```python
from build123d import *

# Parameters (mm, degrees)
SKETCH2_R          = 2
CUT_EXTRUDE1_DEPTH = 41.551456831


with BuildPart() as part:
    # Sketch1 → Revolve1 (revolve)
    with BuildSketch(Plane.XY, mode=Mode.PRIVATE) as revolve1_sk:
        with BuildLine():
            ThreePointArc((5, -39.32455532), (3.535533906, -35.789021414), (0, -34.32455532))
            Line((0, -34.32455532), (0, -30))
            Line((0, -30), (0, 0))
            Line((0, 0), (4, 0))
            Line((4, 0), (4, -3))
            Line((4, -3), (3, -3))
            Line((3, -3), (3, -33))
            ThreePointArc((3, -33), (5.916079783, -35.582897934), (7, -39.32455532))
            Line((7, -39.32455532), (5, -39.32455532))
        make_face()
    revolve(revolve1_sk.sketch.rotate(Axis((0, 0, 0), (0, -1, 0)), 180), axis=Axis((0, 0, 0), (0, -1, 0)))

    # Sketch2 → Cut-Extrude1 (cut, through all)
    with BuildSketch(Plane(origin=(0, 0, 0), x_dir=(1, 0, 0), z_dir=(0, 1, 0))):
        with Locations(Location((0, 0, 0), (0, 0, 180))):
            Circle(SKETCH2_R)
    extrude(amount=-CUT_EXTRUDE1_DEPTH, mode=Mode.SUBTRACT)


solid = part.part
```
Verification items for the finished model (mm, model axes). A direction names the side the tool comes from. Round coordinates to 2 decimals unless told otherwise and drop trailing zeros. Order: outer loops, then holes, each group sorted by start corner. A loop starts at its lowest first (then second) coordinate and runs counter-clockwise, first axis right, second up.
1) Cross-section at A-A, the plane z = 0. Record the cut outline in (x, y), plus the area to 3 significant figures.
Geometry says:
outline: (-7, -39.32) - (-5, -39.32) arc R5 cw to (-2, -34.74) - (-2, 0) - (-4, 0) - (-4, -3) - (-3, -3) - (-3, -33) arc R7 ccw to start; (2, -34.74) arc R5 cw to (5, -39.32) - (7, -39.32) arc R7 ccw to (3, -33) - (3, -3) - (4, -3) - (4, 0) - (2, 0) - close
area: 101 mm2
2) Material ranges on line 1 (Z direction, x = 0, y = -12.5); line 2 (Z direction, x = -2.5, y = -35.5); line 3 (X direction, y = -35.5, z = 1), recorded low to high.
Geometry says:
line 1: z = -3 to -2, 2 to 3
line 2: z = -5.3 to -2.03, 2.03 to 5.3
line 3: x = -5.78 to -3.06, 3.06 to 5.78
3) Cross-section at D-D, the plane z = -5.5. Record the cut outline in (x, y).
Geometry says:
outline: (-4.33, -39.32) - (4.33, -39.32) arc R4.33 ccw to start
4) Draft check along Y on faces 1 (the cylindrical face through (0, -17, -2)), 2 (the cylindrical face through (-2.86, -18.21, -0.9)), 3 (the flat face through (1, 0, -2)). Enter one of: +Y half, -Y half, draft (parallel to the pull), parting line (faces both ways), or undercut.
Geometry says:
face 1: draft
face 2: undercut
face 3: +Y half
5) Depth check by flat-ended pin: pin 1 (2.5 mm diameter, centred on x = 0, z = 2, fed in from -Y); pin 2 (6 mm diameter, centred on x = 5, y = -24.5, fed in from +Z); pin 3 (1 mm diameter, centred on x = -2.5, y = -35.5, fed in from -Z). Enter the tip coordinate at first touch or a pass-through.
Geometry says:
pin 1: stops at y = -35.52
pin 2: stops at z = 2.24
pin 3: stops at z = -5.7
6) Cross-section at C-C, the plane y = -5.5. Record the cut outline in (x, z).
Geometry says:
outline: circle Ø6 at (0, 0); hole circle Ø4 at (0, 0)
7) Tool access check on faces 4 (the flat face through (2, -39.325, -5)), 5 (the flat face through (-1, -3, -3)), 6 (the cylindrical face through (0.867, -1.521, 3.905)). Record the directions out of +Z, -Z, +X, -X, +Y, -Y that give a thin tool (end or side, any length) a straight path to the whole face; none if there is none.
Geometry says:
face 4: +Z, -Z, +X, -X, -Y
face 5: none
face 6: +Y
8) Cross-section at B-B, the plane x = 0. Record the cut outline in (y, z).
Geometry says:
outline: (-39.32, -7) arc R7 ccw to (-33, -3) - (-3, -3) - (-3, -4) - (0, -4) - (0, -2) - (-34.74, -2) arc R5 cw to (-39.32, -5) - close; (-39.32, 5) arc R5 cw to (-34.74, 2) - (0, 2) - (0, 4) - (-3, 4) - (-3, 3) - (-33, 3) arc R7 ccw to (-39.32, 7) - close
